from build123d import *

# Parameters (mm, degrees)
F2_R     = 11.052767
F3_DEPTH = 25.4


with BuildPart() as f1:
    # F0 (on Front) → F1 (revolve)
    with BuildSketch(Plane.XZ):
        Polygon((14.100123, 39.021272), (8.634958, 37.709631), (-26.560698, -10.821025), (-38.802665, -10.821025), (-38.802665, -20.439714), (-26.560698, -20.439714), (-26.560698, -15.411762), align=None)
    revolve(axis=Axis((-38.802665, 0, -15.63037), (0, 0, -1)))

    # F2 (on face) → F3 (cut)
    with BuildSketch(Plane(origin=(0, 0, -20.439714), x_dir=(1, 0, 0), z_dir=(0, 0, -1))):
        with Locations((-38.802665, 0)):
            Circle(F2_R)
    extrude(amount=-F3_DEPTH, mode=Mode.SUBTRACT)


solid = f1.part
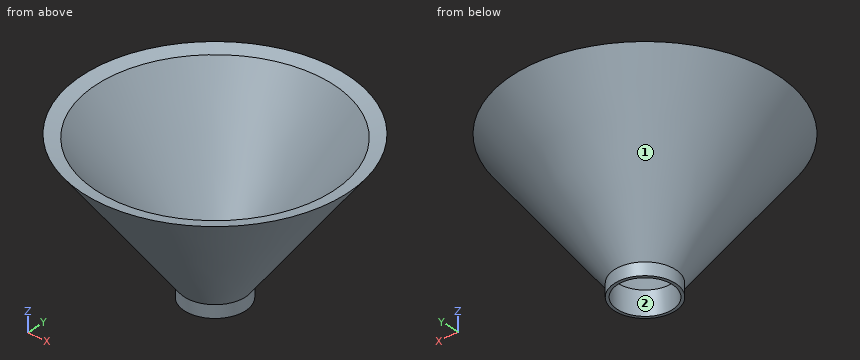
CAD build for the part. Positions are in the model's coordinates, mm. Face numbers are marked on the shaded views. Give positions to 0.01 mm unless a question says otherwise; leave off trailing zeros. Loops run counter-clockwise (first coordinate to the right, second up) from the corner with the lowest first, then second, coordinate; pieces in that order, holes last. Notation, with made-up numbers: M 37,3.5 L 55,3.5 A9 cw 55,7.5 Z; hole C 3.5,5.25 d1. An arc over 180 degrees is marked long. Answer in a Markdown table with one row per item. Add a question column.
Item 1: Band-saw the part on C-C on z = 23. Give the cut face in (x, y).
Item 2: Probe probe 1 along X at (y, z) = (0, -17); probe 2 along X at (y, z) = (35.5, 29.5); probe 3 along Y at (x, z) = (-60, 18.5). List the from-to ranges inside material, lowest first.
Item 3: Band-saw the part on A-A on y = 0. Give the cut face in (x, z).
Item 4: Mould opens along X. For the marked faces 1 and 2 say: +X half, -X half, draft (parallel to the pull), parting line (faces both ways), or undercut.
Item 5: Drop flat-ended pins along their axis: P1, Ø3, axis at x = -49.5, z = -8.5, coming from the -Y side; P2, Ø5, axis at x = -47, y = -24.5, coming from the -Z side; P3, Ø12, axis at x = -64.5, y = -6.5, coming from the -Z side; P4, Ø7.5, axis at x = -35, y = 4.5, coming from the +Z side. Give the stop position or say it passes through.
Item 6: Band-saw the part on B-B on z = -13. Give the cut face in (x, y), then the cut area to 3 significant figures.
Reply:
| question | item | result |
|---|---|---|
| 1 | outline | C -38.8,0 d81.87; hole C -38.8,0 d73.54 |
| 2 | probe 1 | x = -51.04 to -49.86, -27.75 to -26.56 |
| 2 | probe 2 | x = -67.73 to -60.27, -17.34 to -9.88 |
| 2 | probe 3 | y = -31.02 to -25.95, 25.95 to 31.02 |
| 3 | outline | M -91.71,39.02 L -51.04,-15.41 L -51.04,-20.44 L -49.86,-20.44 L -49.86,-10.82 L -51.04,-10.82 L -86.24,37.71 Z; M -27.75,-20.44 L -26.56,-20.44 L -26.56,-15.41 L 14.1,39.02 L 8.63,37.71 L -26.56,-10.82 L -27.75,-10.82 Z |
| 4 | face 1 | parting line |
| 4 | face 2 | undercut |
| 5 | P1 | stops at y = -15.46 |
| 5 | P2 | stops at z = -0.56 |
| 5 | P3 | stops at z = -4.35 |
| 5 | P4 | passes through |
| 6 | outline | C -38.8,0 d28.09; hole C -38.8,0 d22.11 |
| 6 | area | 236 mm^2 |
